from build123d import *

# Parameters (mm, degrees)
SKETCH1_W           = 25.4
SKETCH1_H           = 15.875
BOSS_EXTRUDE1_DEPTH = 38.1
SKETCH2_W           = 8.763
SKETCH2_H           = 25.4
CUT_EXTRUDE1_DEPTH  = 44.184668865
SKETCH3_R           = 1.524
CUT_EXTRUDE2_DEPTH  = 47.473367709
SKETCH4_R           = 2.0955
CUT_EXTRUDE3_DEPTH  = 41.937805342


with BuildPart() as part:
    # Sketch1 → Boss-Extrude1 (new body)
    with BuildSketch(Plane(origin=(0, 0, 0), x_dir=(1, 0, 0), z_dir=(0, 1, 0))):
        Rectangle(SKETCH1_W, SKETCH1_H)
    extrude(amount=BOSS_EXTRUDE1_DEPTH)

    # Sketch2 → Cut-Extrude1 (cut, through all)
    with BuildSketch(Plane.XY.offset(7.9375)):
        with Locations((0, 25.4)):
            Rectangle(SKETCH2_W, SKETCH2_H)
    extrude(amount=-CUT_EXTRUDE1_DEPTH, mode=Mode.SUBTRACT)

    # Sketch3 → Cut-Extrude2 (cut, through all)
    with BuildSketch(Plane(origin=(12.7, 0, 0), x_dir=(0, 0, -1), z_dir=(1, 0, 0))):
        with Locations((0, 34.29)):
            Circle(SKETCH3_R)
    extrude(amount=-CUT_EXTRUDE2_DEPTH, mode=Mode.SUBTRACT)

    # Sketch4 → Cut-Extrude3 (cut, through all)
    with BuildSketch(Plane.XZ):
        with Locations(Location((0, 0, 0), (0, 0, 270))):
            Circle(SKETCH4_R)
    extrude(amount=-CUT_EXTRUDE3_DEPTH, mode=Mode.SUBTRACT)


solid = part.part
The listing builds one solid part. Answer for the finished solid, in the listing's coordinates (mm). A direction names the side the tool comes from. Round coordinates to 2 decimals unless told otherwise and drop trailing zeros. Order: outer loops, then holes, each group sorted by start corner. A loop starts at its lowest first (then second) coordinate and runs counter-clockwise, first axis right, second up. Notation, with made-up numbers: (-34.5, 53.25) - (7.5, 53.25) arc R17 cw to (7.5, 71.25) - close; hole circle Ø5 at (-5, 39). An arc over 180 degrees is marked (long way). Write item = value, one per line. Start each with the question number.
1) Section A-A, the plane y = 34.29 is taken. Write down the section's boundary in (x, z).
2) Section C-C, the plane x = 0 is taken. Write down the section's boundary in (y, z), plus the area to 3 significant figures.
3) For a pull along Y with two mould halves and no side action, classify faces 1 (the cylindrical face through (-8.5, 35.8, 0.2)), 2 (the flat face through (-2, 12.7, 2)), 3 (the flat face through (3, 0, 0)) as released by +Y, released by -Y, zero draft, split by the parting line, or undercut.
4) Section B-B, the plane z = 0 is taken. Write down the section's boundary in (x, y).
5) Straight lines are drawn through the part: L1, parallel to X at y = 32.5, z = -6; L2, parallel to X at y = 7, z = 0; L3, parallel to Y at x = -5.75, z = 0. For each, find the intervals that lie inside material, in ascending order.
6) For faces 4 (the flat face through (-4.382, 25, 0)), 5 (the flat face through (12.7, 19, 0)), determine the directions among +Z, -Z, +X, -X, +Y, -Y from which every point of the face is accessible in a straight line to the end or side of a thin tool.
7) Section D-D, the plane y = 18 is taken. Write down the section's boundary in (x, z).
Results list:
q1.outline = (-12.7, -7.94) - (-4.38, -7.94) - (-4.38, -1.52) - (-12.7, -1.52) - close; (-12.7, 1.52) - (-4.38, 1.52) - (-4.38, 7.94) - (-12.7, 7.94) - close; (4.38, -7.94) - (12.7, -7.94) - (12.7, -1.52) - (4.38, -1.52) - close; (4.38, 1.52) - (12.7, 1.52) - (12.7, 7.94) - (4.38, 7.94) - close
q2.outline = (0, -7.94) - (12.7, -7.94) - (12.7, -2.1) - (0, -2.1) - close; (0, 2.1) - (12.7, 2.1) - (12.7, 7.94) - (0, 7.94) - close
q2.area = 148 mm^2
q3.face_1 = undercut
q3.face_2 = released by +Y
q3.face_3 = released by -Y
q4.outline = (-12.7, 0) - (-2.1, 0) - (-2.1, 12.7) - (-4.38, 12.7) - (-4.38, 32.77) - (-12.7, 32.77) - close; (-12.7, 35.81) - (-4.38, 35.81) - (-4.38, 38.1) - (-12.7, 38.1) - close; (2.1, 0) - (12.7, 0) - (12.7, 32.77) - (4.38, 32.77) - (4.38, 12.7) - (2.1, 12.7) - close; (4.38, 35.81) - (12.7, 35.81) - (12.7, 38.1) - (4.38, 38.1) - close
q5.L1 = -12.7 to -4.38, 4.38 to 12.7
q5.L2 = -12.7 to -2.1, 2.1 to 12.7
q5.L3 = 0 to 32.77, 35.81 to 38.1
q6.face_4 = +Z, -Z, +Y
q6.face_5 = +Z, -Z, +X, +Y, -Y
q7.outline = (-12.7, -7.94) - (-4.38, -7.94) - (-4.38, 7.94) - (-12.7, 7.94) - close; (4.38, -7.94) - (12.7, -7.94) - (12.7, 7.94) - (4.38, 7.94) - close
